Check sheet for the drawn part. Datum: minimum x, y, z corner. Units: mm. A direction names the side the tool comes from. Round coordinates to 2 decimals unless told otherwise and drop trailing zeros. Write each loop counter-clockwise with the first axis right and the second up, starting at its lowest first coordinate (ties: lowest second). Pieces come first, ordered by that corner, then holes. Notation, with made-up numbers: (85.25, 54) - (131.25, 54) arc R21 cw to (131.25, 76) - close; hole circle Ø1 at (62, 2). An arc over 180 degrees is marked (long way). Answer as a JSON object with one key per item and string values.
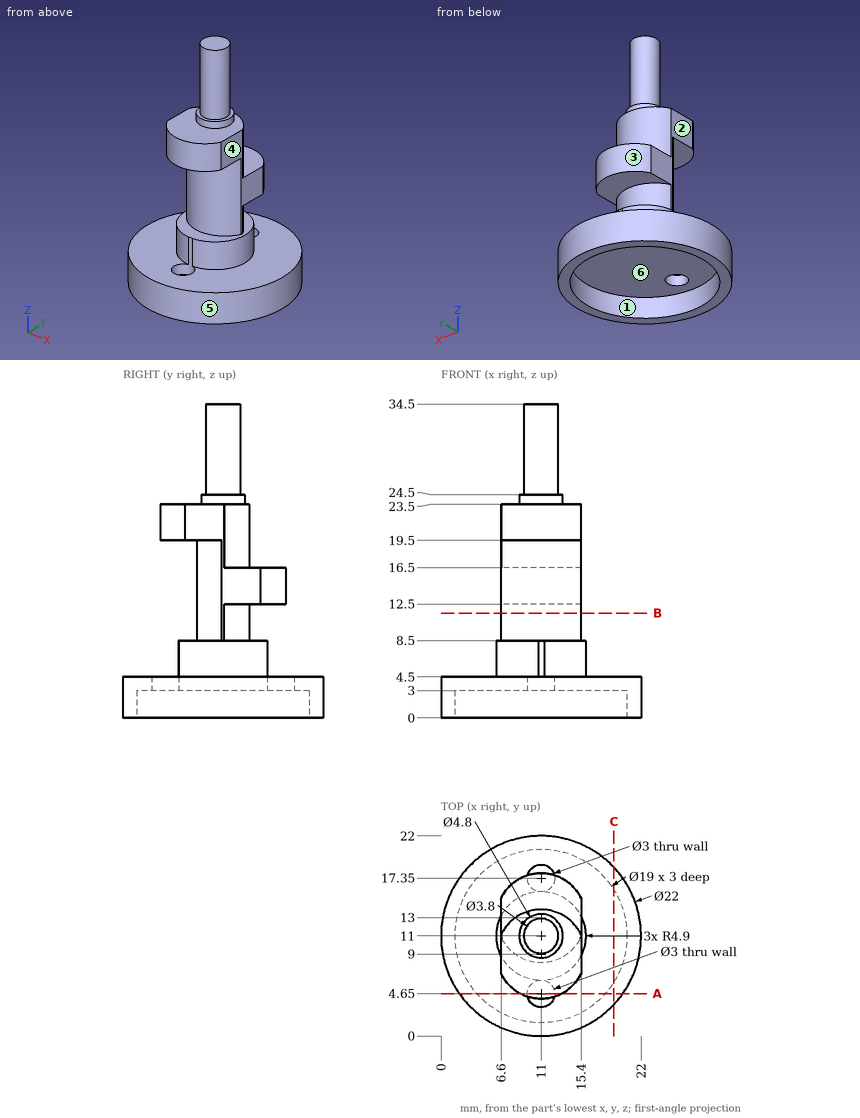
Q1. Release check for a two-part mould opening along Y. For the marked faces 4, 5 and 6 record: released by +Y, released by -Y, zero draft, split by the parting line, or undercut.
Geometry check:
{"face 4": "zero draft", "face 5": "split by the parting line", "face 6": "undercut"}
Q2. Gauge pin test, flat ends, axial feed: P1, Ø1.5, axis at x = 14.5, y = 14, coming from the -Z side; P2, Ø4, axis at y = 13.5, z = 20.5, coming from the +X side; P3, Ø2, axis at y = 9.5, z = 30.5, coming from the +X side. Record the tip position at first contact, or that the pin passes through.
Geometry check:
{"P1": "stops at z = 3", "P2": "stops at x = 15.21", "P3": "stops at x = 12.83"}
Q3. Section check A-A, the plane y = 4.65. Record the cut outline in (x, z).
Geometry check:
{"outline": "(2.02, 0) - (3.93, 0) - (3.93, 3) - (9.5, 3) - (9.5, 4.5) - (2.02, 4.5) - close; (8.74, 19.5) - (13.26, 19.5) - (13.26, 23.5) - (8.74, 23.5) - close; (12.5, 3) - (18.07, 3) - (18.07, 0) - (19.98, 0) - (19.98, 4.5) - (12.5, 4.5) - close"}
Q4. Section check C-C, the plane x = 19. Record the cut outline in (y, z).
Geometry check:
{"outline": "(3.45, 0) - (5.88, 0) - (5.88, 3) - (16.12, 3) - (16.12, 0) - (18.55, 0) - (18.55, 4.5) - (3.45, 4.5) - close"}
Q5. Material ranges on line 1 along Y through (x, z) = (11, 2.15); line 2 along Z through (x, y) = (14.75, 18); line 3 along Z through (x, y) = (7, 20.5), recorded low to high. Write a range as [from, to].
Geometry check:
{"line 1": "y = [0, 1.5], [20.5, 22]", "line 2": "z = [3, 4.5]", "line 3": "z = [0, 4.5]"}
Q6. Set-up check for the marked faces 1, 2 and 3: record each of +Z, -Z, +X, -X, +Y, -Y from which the full face is reachable in a straight line by a thin tool's end or side.
Geometry check:
{"face 1": "-Z", "face 2": "+Z, -X, +Y, -Y", "face 3": "+Z, +Y"}
Q7. Section check B-B, the plane z = 11.5. Record the cut outline in (x, y), then the cut area to 3 significant figures.
Geometry check:
{"outline": "(6.6, 10.84) arc R4.9 ccw to (15.4, 10.84) - (15.4, 11.16) arc R4.9 ccw to (6.6, 11.16) - close", "area": "37.3 mm2"}
